from build123d import *

# Parameters (mm, degrees)
SKETCH3_R          = 2.525
CUT_EXTRUDE1_DEPTH = 4
SKETCH6_R          = 3
CUT_EXTRUDE4_DEPTH = 11
SKETCH7_R          = 3.3
CUT_EXTRUDE5_DEPTH = 10
SKETCH9_R          = 1
CUT_EXTRUDE7_DEPTH = 2
CUT_EXTRUDE8_REACH = 117.07
SKETCH10_R         = 3.3
CHAMFER1_SIZE      = 0.5


with BuildPart() as part:
    # Sketch2 → Revolve1 (revolve)
    with BuildSketch(Plane.XY, mode=Mode.PRIVATE) as revolve1_sk:
        Polygon((0, 80), (0, 52.5), (11, 52.5), (11, 32.5), (18, 32.5), (18, 29.5), (21, 29.5), (21, 80), align=None)
    revolve(revolve1_sk.sketch.rotate(Axis((0, 0, 0), (1, 0, 0)), 90), axis=Axis((0, 0, 0), (1, 0, 0)))

    # Sketch3 → Cut-Extrude1 (cut)
    with BuildSketch(Plane.ZY):
        with Locations((0, 60)):
            Circle(SKETCH3_R)
        with Locations((12.077911205, 58.771796475)):
            Circle(SKETCH3_R)
        with Locations((23.661351307, 55.137468697)):
            Circle(SKETCH3_R)
        with Locations((34.276092906, 49.245806472)):
            Circle(SKETCH3_R)
        with Locations((43.487567234, 41.338015145)):
            Circle(SKETCH3_R)
        with Locations((50.91865545, 31.73784062)):
            Circle(SKETCH3_R)
        with Locations((56.265127929, 20.838315171)):
            Circle(SKETCH3_R)
        with Locations((59.30809946, 9.08566665)):
            Circle(SKETCH3_R)
        with Locations((59.92299043, -3.03895013)):
            Circle(SKETCH3_R)
        with Locations((58.084627132, -15.039151936)):
            Circle(SKETCH3_R)
        with Locations((53.868272374, -26.423649093)):
            Circle(SKETCH3_R)
        with Locations((47.446544216, -36.726358953)):
            Circle(SKETCH3_R)
        with Locations((39.082348963, -45.525487362)):
            Circle(SKETCH3_R)
        with Locations((29.118117752, -52.460796969)):
            Circle(SKETCH3_R)
        with Locations((17.961787378, -57.248355384)):
            Circle(SKETCH3_R)
        with Locations((6.070099319, -59.692159404)):
            Circle(SKETCH3_R)
        with Locations((-6.070099319, -59.692159404)):
            Circle(SKETCH3_R)
        with Locations((-17.961787378, -57.248355384)):
            Circle(SKETCH3_R)
        with Locations((-29.118117752, -52.460796969)):
            Circle(SKETCH3_R)
        with Locations((-39.082348963, -45.525487362)):
            Circle(SKETCH3_R)
        with Locations((-47.446544216, -36.726358953)):
            Circle(SKETCH3_R)
        with Locations((-53.868272374, -26.423649093)):
            Circle(SKETCH3_R)
        with Locations((-58.084627132, -15.039151936)):
            Circle(SKETCH3_R)
        with Locations((-59.92299043, -3.03895013)):
            Circle(SKETCH3_R)
        with Locations((-59.30809946, 9.08566665)):
            Circle(SKETCH3_R)
        with Locations((-56.265127929, 20.838315171)):
            Circle(SKETCH3_R)
        with Locations((-50.91865545, 31.73784062)):
            Circle(SKETCH3_R)
        with Locations((-43.487567234, 41.338015145)):
            Circle(SKETCH3_R)
        with Locations((-34.276092906, 49.245806472)):
            Circle(SKETCH3_R)
        with Locations((-23.661351307, 55.137468697)):
            Circle(SKETCH3_R)
        with Locations((-12.077911205, 58.771796475)):
            Circle(SKETCH3_R)
    extrude(amount=-CUT_EXTRUDE1_DEPTH, mode=Mode.SUBTRACT)

    # Sketch6 → Cut-Extrude4 (cut)
    with BuildSketch(Plane.ZY):
        with Locations((53.875586653, 44.692517973)):
            Circle(SKETCH6_R)
        with Locations((69.69817519, -6.493410136)):
            Circle(SKETCH6_R)
        with Locations((44.692517973, -53.875586653)):
            Circle(SKETCH6_R)
        with Locations((-6.493410136, -69.69817519)):
            Circle(SKETCH6_R)
        with Locations((-53.875586653, -44.692517973)):
            Circle(SKETCH6_R)
        with Locations((-69.69817519, 6.493410136)):
            Circle(SKETCH6_R)
        with Locations((-44.692517973, 53.875586653)):
            Circle(SKETCH6_R)
        with Locations((6.493410136, 69.69817519)):
            Circle(SKETCH6_R)
    extrude(amount=-CUT_EXTRUDE4_DEPTH, mode=Mode.SUBTRACT)

    # Sketch7 → Cut-Extrude5 (cut)
    with BuildSketch(Plane.ZY.offset(-21)):
        with Locations((53.875586653, 44.692517973)):
            Circle(SKETCH7_R)
        with Locations((69.69817519, -6.493410136)):
            Circle(SKETCH7_R)
        with Locations((44.692517973, -53.875586653)):
            Circle(SKETCH7_R)
        with Locations((-6.493410136, -69.69817519)):
            Circle(SKETCH7_R)
        with Locations((-53.875586653, -44.692517973)):
            Circle(SKETCH7_R)
        with Locations((-69.69817519, 6.493410136)):
            Circle(SKETCH7_R)
        with Locations((-44.692517973, 53.875586653)):
            Circle(SKETCH7_R)
        with Locations((6.493410136, 69.69817519)):
            Circle(SKETCH7_R)
    extrude(amount=CUT_EXTRUDE5_DEPTH, mode=Mode.SUBTRACT)

    # Sketch9 → Cut-Extrude7 (cut)
    with BuildSketch(Plane.ZY):
        with Locations((2.51770285, -71.46627686)):
            Circle(SKETCH9_R)
    extrude(amount=-CUT_EXTRUDE7_DEPTH, mode=Mode.SUBTRACT)

    # Sketch10 → Cut-Extrude8 (cut, up to next)
    with BuildSketch(Plane(origin=(21, 0, 0), x_dir=(0, 0, -1), z_dir=(1, 0, 0)), mode=Mode.PRIVATE) as cut_extrude8_sk1:
        with Locations((23.431880753, 37.241736861)):
            Circle(SKETCH10_R)
    cut_extrude8_tool1 = extrude(cut_extrude8_sk1.sketch, amount=-CUT_EXTRUDE8_REACH, mode=Mode.PRIVATE) & part.part
    # Sketch10 → Cut-Extrude8 (cut, up to next)
    with BuildSketch(Plane(origin=(21, 0, 0), x_dir=(0, 0, -1), z_dir=(1, 0, 0)), mode=Mode.PRIVATE) as cut_extrude8_sk2:
        with Locations((20.536349826, -38.913472421)):
            Circle(SKETCH10_R)
    cut_extrude8_tool2 = extrude(cut_extrude8_sk2.sketch, amount=-CUT_EXTRUDE8_REACH, mode=Mode.PRIVATE) & part.part
    # Sketch10 → Cut-Extrude8 (cut, up to next)
    with BuildSketch(Plane(origin=(21, 0, 0), x_dir=(0, 0, -1), z_dir=(1, 0, 0)), mode=Mode.PRIVATE) as cut_extrude8_sk3:
        with Locations((-43.968230579, 1.67173556)):
            Circle(SKETCH10_R)
    cut_extrude8_tool3 = extrude(cut_extrude8_sk3.sketch, amount=-CUT_EXTRUDE8_REACH, mode=Mode.PRIVATE) & part.part
    add(cut_extrude8_tool1.solids().sort_by_distance((21, 37.241737, -23.431881))[0], mode=Mode.SUBTRACT)
    add(cut_extrude8_tool2.solids().sort_by_distance((21, -38.913472, -20.53635))[0], mode=Mode.SUBTRACT)
    add(cut_extrude8_tool3.solids().sort_by_distance((21, 1.671736, 43.968231))[0], mode=Mode.SUBTRACT)

    # Chamfer1
    chamfer1_edges = [part.edges().sort_by_distance(p)[0] for p in [
        (21, -6.493410136, 66.39817519),
        (21, -53.875586653, 41.392517973),
        (21, -69.69817519, -9.793410136),
        (21, -44.692517973, -57.175586653),
        (21, 6.493410136, -72.99817519),
        (21, 44.692517973, 50.575586653),
        (21, 37.241736861, -20.131880753),
        (21, -38.913472421, -17.236349826),
        (21, 1.67173556, 47.268230579),
    ]]
    chamfer(chamfer1_edges, length=CHAMFER1_SIZE)


solid = part.part
The model under review builds one solid part; all positions refer to its coordinate system, in mm. A direction names the side the tool comes from. Round coordinates to 2 decimals unless told otherwise and drop trailing zeros. Answer as a JSON object with one key per item and string values.
Item 1: The part is to be moulded in two halves that separate along Z. For faces 3 (the face through (16.07, 57.148, -45.122)), 4 (the face through (0, 17, 52)), say which applies: +Z half, -Z half, draft (parallel to the pull), parting line (faces both ways), or undercut.
Check sheet entries:
{"face 3": "undercut", "face 4": "draft"}
Item 2: For line 1 along Y through (x, z) = (16.5, 0); line 2 along Y through (x, z) = (8.75, -42); line 3 along Y through (x, z) = (14.75, -25), list the stretches that pass through material, from the lowest coordinate up.
Check sheet entries:
{"line 1": "-80 to -32.5, 32.5 to 80", "line 2": "-68.09 to -31.5, 31.5 to 52.55, 55.2 to 68.09", "line 3": "-75.99 to -20.77, 20.77 to 34.34, 40.15 to 75.99"}
Item 3: Clearance check with flat-ended pins moving along their axes: P1, Ø6, axis at x = 17, y = -19, coming from the +Z side; P2, Ø2.5, axis at y = 54, z = -24, coming from the -X side; P3, Ø6, axis at y = 41.34, z = -43.49, coming from the -X side; P4, Ø3, axis at x = 12.5, y = -16.5, coming from the +Z side. State where each tip first meets the part, or that it passes through.
Check sheet entries:
{"P1": "z = 78.38", "P2": "x = 4", "P3": "x = 0", "P4": "z = 78.58"}
Item 4: Tool access review of faces 1 (the face through (15.817, 6.639, -72.995)), 2 (the face through (4, 49, 34)): name each direction out of +Z, -Z, +X, -X, +Y, -Y from which nothing blocks a thin tool from reaching the whole face with its end or side.
Check sheet entries:
{"face 1": "+X", "face 2": "-X"}
Item 5: We need section A-A, the plane x = 6. State how many separate pieces and enclosed holes the cut face has, and give its area (3 significant figures).
Check sheet entries:
{"separate pieces": "1", "enclosed holes": "9", "area": "11,200 mm2"}
